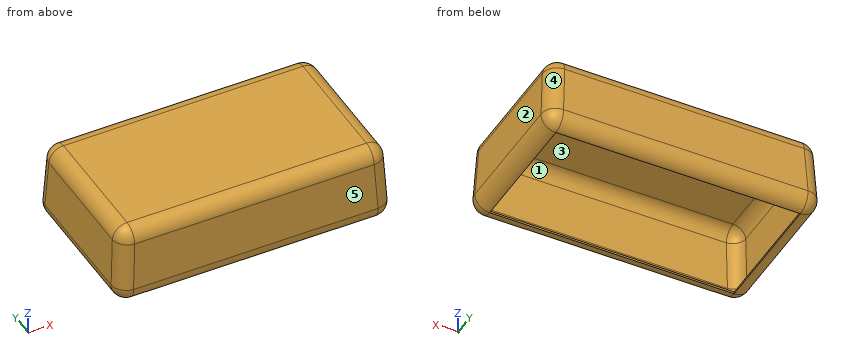
```python
from build123d import *

# Parameters (mm, degrees)
F0_W     = 177.8
F0_H     = 101.6
F1_DEPTH = 50.8
F1_TAPER = 3
F2_R     = 9.525
F3_T     = -1.27


# Not quite as in the source:
# - a shell that OpenCascade refuses in one call is made with other operations: the cavity is built on its own and cut out


with BuildPart() as f1:
    # F0 (on Top) → F1 (new body)
    with BuildSketch(Plane.XY):
        Rectangle(F0_W, F0_H)
    extrude(amount=F1_DEPTH, taper=F1_TAPER)

    # F2
    f2_edges = [f1.edges().sort_by_distance(p)[0] for p in [
        (0, -50.8, 0),
        (87.568842, -49.468842, 25.4),
        (-87.568842, -49.468842, 25.4),
        (0, -48.137685, 50.8),
        (0, 48.137685, 50.8),
        (-86.237685, 0, 50.8),
        (86.237685, 0, 50.8),
        (88.9, 0, 0),
        (87.568842, 49.468842, 25.4),
        (0, 50.8, 0),
        (-87.568842, 49.468842, 25.4),
        (-88.9, 0, 0),
    ]]
    fillet(f2_edges, radius=F2_R)

    # F3: a shell. OpenCascade refuses it in one call, so the cavity is built on its own and cut out:
    # the body offset inwards by the wall thickness, plus a prism from it out through each open face.
    f3_core = offset(f1.part, amount=F3_T, mode=Mode.PRIVATE)
    f3_exits = [f3_core.faces().sort_by_distance(p)[0] for p in [
        (0, 0, 1.27),
    ]]
    add(f3_core, mode=Mode.SUBTRACT)
    extrude(f3_exits, amount=-F3_T, mode=Mode.SUBTRACT)


solid = f1.part
```
Work out the finished part from the listing and answer in its coordinate system (mm). Face numbers are marked on the shaded views. A direction names the side the tool comes from. Coordinates: 2 decimals unless noted, no trailing zeros. Loops run counter-clockwise (first coordinate to the right, second up) from the corner with the lowest first, then second, coordinate; pieces in that order, holes last. Notation, with made-up numbers: (-16.5, -7.75) -> (-9.5, -7.75) arc R17 ccw to (-9.5, 11.25) -> close; hole circle Ø7 at (44, -10). An arc over 180 degrees is marked (long way). Answer as CSV lines item,"result".
Q1. Each of these flat-tipped pins is pushed along its axis until it touches: pin 1 (1.4 mm diameter, centred on x = -38, z = 1, fed in from +Y); pin 2 (23.5 mm diameter, centred on x = 22, y = 8.5, fed in from -Z); pin 3 (3 mm diameter, centred on x = 44, z = 44, fed in from -Y). Where does it stop, or does it pass through?
Findings:
pin 1,"stops at y = 46.19"
pin 2,"stops at z = 49.53"
pin 3,"stops at y = -48.54"
Q2. For a pull along X with two mould halves and no side action, classify the marked faces 3, 4 and 5 as +X half, -X half, draft (parallel to the pull), parting line (faces both ways), or undercut.
Findings:
face 3,"undercut"
face 4,"+X half"
face 5,"draft"
Q3. Find the intervals of material crossed by probe 1 along Y at (x, z) = (36, 42); probe 2 along X at (y, z) = (26.5, 9); probe 3 along Z at (x, y) = (65.5, 35.5), in increasing order.
Findings:
probe 1,"y = -48.6 to -47.32, 47.32 to 48.6"
probe 2,"x = -88.37 to -87.1, 87.1 to 88.37"
probe 3,"z = 49.53 to 50.8"
Q4. A tool of negligible diameter and unlimited length cuts with its end or side. For the marked faces 1 and 2, from which of +Z, -Z, +X, -X, +Y, -Y can it reach the whole face along a straight path? Write none if from no direction.
Findings:
face 1,"none"
face 2,"+Z, +X, +Y, -Y"
Q5. The part is cut by section C-C on z = 6. Write down the section's boundary in (x, y).
Findings:
outline,"(-87.71, -40.76) arc R8.85 ccw to (-78.86, -49.61) -> (78.86, -49.61) arc R8.85 ccw to (87.71, -40.76) -> (87.71, 40.76) arc R8.85 ccw to (78.86, 49.61) -> (-78.86, 49.61) arc R8.85 ccw to (-87.71, 40.76) -> close; hole (-86.33, -40.76) arc R7.46 ccw to (-78.86, -48.23) -> (78.86, -48.23) arc R7.46 ccw to (86.33, -40.76) -> (86.33, 40.76) arc R7.46 ccw to (78.86, 48.23) -> (-78.86, 48.23) arc R7.46 ccw to (-86.33, 40.76) -> close"
Q6. The part is cut by section D-D on z = 44.5. Write down the section's boundary in (x, y).
Findings:
outline,"(-86.16, -39.1) arc R8.96 ccw to (-77.2, -48.06) -> (77.2, -48.06) arc R8.96 ccw to (86.16, -39.1) -> (86.16, 39.1) arc R8.96 ccw to (77.2, 48.06) -> (-77.2, 48.06) arc R8.96 ccw to (-86.16, 39.1) -> close; hole (-84.8, -39.1) arc R7.6 ccw to (-77.2, -46.7) -> (77.2, -46.7) arc R7.6 ccw to (84.8, -39.1) -> (84.8, 39.1) arc R7.6 ccw to (77.2, 46.7) -> (-77.2, 46.7) arc R7.6 ccw to (-84.8, 39.1) -> close"
